Autodesk Inventor part; units mm, degrees
ref_plane "Work Plane1" through (33.575, 0, 0) normal (0, 0, -1) x (1, 0, 0)
ref_plane "YZ Plane" through (0, 0, 0) normal (1, 0, 0) x (0, 1, 0)
ref_plane "XZ Plane" through (0, 0, 0) normal (0, 1, 0) x (-1, 0, 0)
sketch "Sketch1" plane through (0, 0, 0) normal (0, 0, 1) x (1, 0, 0)
  line L0 (0, 0) -> (8, 0)
  line L1 (8, 0) -> (8, 3)
  line L2 (8, 3) -> (5.3, 3)
  line L3 (5.3, 3) -> (4.6866, 2.3866)
  line L4 (4.6866, 2.3866) -> (3.9135, 2.3866)
  line L5 (3.9135, 2.3866) -> (0.65, 5.65)
  line L6 (0.65, 5.65) -> (0, 5.65)
  line L7 (0, 5.65) -> (0, 0)
  line L8 (5.3, 3) -> (3.3, 3) construction
  line L9 (-1.6, 0) -> (9.6, 0)
  line L10 (0, 6.78) -> (0, -1.13)
  dimension "d0" = 8
  dimension "d1" = 45
  dimension "d2" = 0.6135
  dimension "d3" = 2.7
  dimension "d4" = 3.3
  dimension "d5" = 4.7731
  dimension "d6" = 6
  dimension "d7" = 11.3
revolve "Body" add sketch "Sketch1" angle 360 about axis through (0, 0, 0) along (1, 0, 0)
sketch "Sketch2" plane through (0, 0, 0) normal (-1, 0, 0) x (0, 0, 1)
  line L0 (5.65, -0.955) -> (-5.65, -0.955)
  line L1 (-5.65, -0.955) -> (-5.65, 0.955)
  line L2 (-5.65, 0.955) -> (5.65, 0.955)
  line L3 (5.65, 0.955) -> (5.65, -0.955)
  line L4 (0, 0.955) -> (0, -0.955) construction
  line L5 (-5.65, 0) -> (5.65, 0) construction
  line L6 (0, 5.65) -> (0, 0)
  dimension "d15" = 1.91
  dimension "d16" = 11.3
extrude "Slot" cut sketch "Sketch2" against normal blind 1.6
thread "Thread"
chamfer "Chamfer1" distance 0.6135 distance2 0.3067 1 edges at (8, -3, 0) measured on face at (8, 0.7485, -0.6631)
ref_plane "Work Plane1" through (33.575, 0, 0) normal (0, 0, -1) x (1, 0, 0)
equation "\"d15\" = SBR"
equation "\"d16\" = KOD"
equation "\"d8\" = STI"
equation "\"d10\" = GEL"
equation "\"d12\" = -0.5 * SPD + 0.5 * GD"
equation "\"d13\" = 0.5 * GAL"
equation "\"d0\" = NLG"
equation "\"d1\" = 0.5 * SEWI"
equation "\"d2\" = GAL"
equation "\"d3\" = GEL"
equation "\"d4\" = KOH"
equation "\"d5\" = BDM"
equation "\"d6\" = GD"
equation "\"d7\" = KOD"
equation "\"NLG\" = 8"
equation "\"GAL\" = 0.61345 * PTC"
equation "\"GEL\" = 2.7"
equation "\"KOH\" = 3.3"
equation "\"KOD\" = 11.3"
equation "\"SEWI\" = 90deg"
equation "\"BDM\" = NND - 1.2269 * PTC"
equation "\"GD\" = NND"
equation "\"SBR\" = 1.91"
equation "\"STI\" = 1.6"
equation "\"SPD\" = NND - 1.2269 * PTC"
equation "\"GUL\" = 0.61345 * PTC"
equation "\"PTC\" = 1"
equation "\"EPV\" = 6.3"
equation "\"THREADDIA\" = 6"
equation "\"TOA\" = 30deg"
equation "\"NND\" = 6"
equation "\"GD1\" = THREADDIA - 1.2269 * PTC"
properties part number "ISO 2009 - M6 x 8" material "Stainless Steel, 440C"
Part model, mm, in its own coordinate system. A direction names the side the tool comes from. Coordinates: 2 decimals unless noted, no trailing zeros. Write each loop counter-clockwise with the first axis right and the second up, starting at its lowest first coordinate (ties: lowest second). Pieces come first, ordered by that corner, then holes. Notation, with made-up numbers: (31.5, 57) - (87.5, 57) arc R31 ccw to (87.5, 92) - close; hole circle Ø2 at (31, 30.5). An arc over 180 degrees is marked (long way). Put each result on its own line as item: value.
1. 3-axis set-ups, long thin cutter, end or side, ignore diameter. For faces 1 (the flat face through (1, 0.955, 0)), 2 (the conical face through (3.71, -0.56, 2.53)), 3 (the cylindrical face through (0.32, -5.65, -0.11)): which of +Z, -Z, +X, -X, +Y, -Y reach the whole face in a straight line?
Final values:
face 1: +Z, -Z, -X
face 2: none
face 3: +X, -X, -Y
2. Band-saw the part on A-A (y = 0). Write the cut outline in (x, z), then the cut area to 3 significant figures.
Final values:
outline: (1.6, -4.7) - (3.91, -2.39) - (4.69, -2.39) - (5.3, -3) - (7.69, -3) - (8, -2.39) - (8, 2.39) - (7.69, 3) - (5.3, 3) - (4.69, 2.39) - (3.91, 2.39) - (1.6, 4.7) - close
area: 39.4 mm²
3. Probe line 1 along Y through (x, z) = (1.5, 3.75) (3 decimals); line 2 along X through (y, z) = (0.5, -2.25); line 3 along X through (y, z) = (-1.5, -2.75). List the from-to ranges inside material, lowest first. Write a range as [from, to].
Final values:
line 1: y = [-2.996, -0.955], [0.955, 2.996]
line 2: x = [1.6, 8]
line 3: x = [0, 3.17]
4. Two-plate mould, pull along Y, no slides. Class faces 4 (the flat face through (1, -0.955, 0)), 5 (the flat face through (0, 3, 0)), 6 (the cylindrical face through (6, -3, 0)): +Y half, -Y half, draft (parallel to the pull), parting line (faces both ways), or undercut.
Final values:
face 4: undercut
face 5: draft
face 6: parting line
5. Flat gauge pins, fed straight in: pin 1 Ø0.6 at (y, z) = (0.5, -1) entering from -X; pin 2 Ø4 at (x, z) = (4, 2.5) entering from +Y; pin 3 Ø1 at (x, z) = (4.5, -3) entering from -Y; pin 4 Ø1 at (x, y) = (4.5, -2.5) entering from +Z. Where does each tip first touch, or does it go through?
Final values:
pin 1: stops at x = 1.6
pin 2: stops at y = 3.77
pin 3: passes through
pin 4: stops at z = 1.39
6. Band-saw the part on D-D (x = 6). Write the cut outline in (y, z).
Final values:
outline: circle Ø6 at (0, 0)
7. Band-saw the part on C-C (x = 5). Write the cut outline in (y, z), then the cut area to 3 significant figures.
Final values:
outline: circle Ø5.4 at (0, 0)
area: 22.9 mm²
